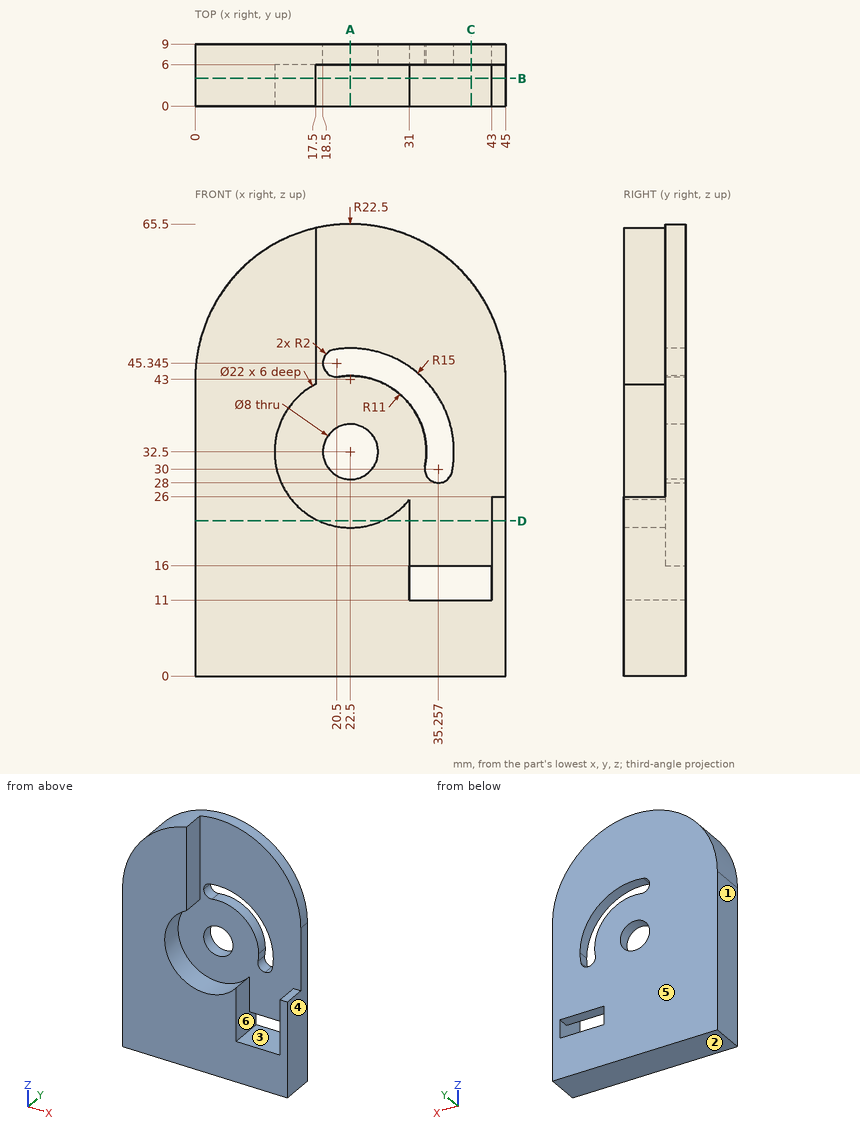
Drawing for the job (mm, zero at the part's lowest x, y, z). A direction names the side the tool comes from. Give positions to 0.01 mm unless a question says otherwise; leave off trailing zeros. Order: outer loops, then holes, each group sorted by start corner. A loop starts at its lowest first (then second) coordinate and runs counter-clockwise, first axis right, second up. Notation, with made-up numbers: M -4.5,53 L 9.5,53 A21 ccw 9.5,58 Z; hole C 63,28 d6. An arc over 180 degrees is marked long. Put each result on its own line as item: value.
Item 1: Slice it at C-C, the plane x = 40. Write the cut outline in (y, z).
From the geometry:
outline: M 0,0 L 9,0 L 9,11 L 0,11 Z; M 6,16 L 9,16 L 9,57.14 L 6,57.14 Z
Item 2: Slice it at A-A, the plane x = 22.5. Write the cut outline in (y, z).
From the geometry:
outline: M 0,0 L 9,0 L 9,28.5 L 6,28.5 L 6,21.5 L 0,21.5 Z; M 6,36.5 L 9,36.5 L 9,43.5 L 6,43.5 Z; M 6,47.5 L 9,47.5 L 9,65.5 L 6,65.5 Z
Item 3: Flat gauge pins, fed straight in: pin 1 Ø1 at (x, y) = (26, 1.5) entering from +Z; pin 2 Ø8 at (x, z) = (9, 13) entering from -Y; pin 3 Ø1.8 at (y, z) = (4.5, 54.5) entering from +X; pin 4 Ø5 at (x, y) = (15.5, 8) entering from +Z (1 decimal). Where does each tip first touch, or does it go through?
From the geometry:
pin 1: stops at z = 22.25
pin 2: stops at y = 0
pin 3: stops at x = 17.5
pin 4: stops at z = 65
Item 4: Slice it at B-B, the plane y = 4. Write the cut outline in (x, z).
From the geometry:
outline: M 0,0 L 45,0 L 45,26 L 43,26 L 43,11 L 31,11 L 31,25.52 A11 cw long 17.5,42.3 L 17.5,64.94 A22.5 ccw 0,43 Z
Item 5: Two-plate mould, pull along X, no slides. Class the marked faces 1, 2, 3 and 4: +X half, -X half, draft (parallel to the pull), parting line (faces both ways), or undercut.
From the geometry:
face 1: -X half
face 2: draft
face 3: undercut
face 4: +X half
Item 6: Probe line 1 (Z direction, x = 22.5, y = 8.3); line 2 (Y direction, x = 23.5, z = 26.5); line 3 (Z direction, x = 33, y = 3.5). List the from-to ranges inside material, lowest first. Write a range as [from, to].
From the geometry:
line 1: z = [0, 28.5], [36.5, 43.5], [47.5, 65.5]
line 2: y = [6, 9]
line 3: z = [0, 11]
Item 7: 3-axis set-ups, long thin cutter, end or side, ignore diameter. For the marked faces 5 and 6: which of +Z, -Z, +X, -X, +Y, -Y reach the whole face in a straight line?
From the geometry:
face 5: +Z, -Z, +X, -X, +Y
face 6: -Y
Item 8: Slice it at D-D, the plane z = 22.5. Write the cut outline in (x, y), plus the area to 3 significant figures.
From the geometry:
outline: M 0,0 L 17.92,0 L 17.92,6 L 27.08,6 L 27.08,0 L 31,0 L 31,6 L 43,6 L 43,0 L 45,0 L 45,9 L 0,9 Z
area: 278 mm2
